```python
from build123d import *

# Parameters (mm, degrees)
BOX044_W               = 4
BOX044_H               = 7
BOX044_DEPTH           = 25
BOX044_PLACEMENT_ANGLE = 45
CYLINDER100_R          = 22
CYLINDER100_DEPTH      = 28
BOX042_W               = 26.5
BOX042_H               = 20.2
BOX042_DEPTH           = 28
BOX042_PLACEMENT_ANGLE = 45
BOX043_W               = 16.5
BOX043_H               = 36
BOX043_DEPTH           = 28
BOX043_PLACEMENT_ANGLE = 45
BOX045_W               = 10
BOX045_H               = 36
BOX045_DEPTH           = 3
BOX045_PLACEMENT_ANGLE = 45


with BuildPart() as cube023:
    # Box044 → Box044 (new body)
    with BuildSketch(Plane.XY):
        with Locations((2, 3.5)):
            Rectangle(BOX044_W, BOX044_H)
    extrude(amount=BOX044_DEPTH)


with BuildPart() as cube023_1:
    # Box044 placement: moved
    add(cube023.part.moved(Location((17, 12, -28))).rotate(Axis((17, 12, -28), (0, 0, 1)), BOX044_PLACEMENT_ANGLE))


with BuildPart() as cylinder100:
    # Cylinder100 → Cylinder100 (new body)
    with BuildSketch(Plane(origin=(7, 7, -28), x_dir=(1, 0, 0), z_dir=(0, 0, 1))):
        Circle(CYLINDER100_R)
    extrude(amount=CYLINDER100_DEPTH)


with BuildPart() as inner001:
    # Box042 → Box042 (new body)
    with BuildSketch(Plane.XY):
        with Locations((13.25, 10.1)):
            Rectangle(BOX042_W, BOX042_H)
    extrude(amount=BOX042_DEPTH)


with BuildPart() as inner001_1:
    # Box042 placement: moved
    add(inner001.part.moved(Location((24.2, 10, -28))).rotate(Axis((24.2, 10, -28), (0, 0, 1)), BOX042_PLACEMENT_ANGLE))


with BuildPart() as cut106:
    # Box043 → Box043 (new body)
    with BuildSketch(Plane.XY):
        with Locations((8.25, 18)):
            Rectangle(BOX043_W, BOX043_H)
    extrude(amount=BOX043_DEPTH)


with BuildPart() as cut106_1:
    # Box043 placement: moved
    add(cut106.part.moved(Location((27.2, 2, -28))).rotate(Axis((27.2, 2, -28), (0, 0, 1)), BOX043_PLACEMENT_ANGLE))

    # Cut105: cut inner001
    add(inner001_1.part, mode=Mode.SUBTRACT)

    # Common007: intersect Cylinder100
    add(cylinder100.part, mode=Mode.INTERSECT)

    # Cut106: cut Cube023
    add(cube023_1.part, mode=Mode.SUBTRACT)


with BuildPart() as fusion030:
    # Box045 → Box045 (new body)
    with BuildSketch(Plane.XY):
        with Locations((5, 18)):
            Rectangle(BOX045_W, BOX045_H)
    extrude(amount=BOX045_DEPTH)


with BuildPart() as fusion030_1:
    # Box045 placement: moved
    add(fusion030.part.moved(Location((20.19, -5, -3))).rotate(Axis((20.19, -5, -3), (0, 0, 1)), BOX045_PLACEMENT_ANGLE))

    # Fusion030: union Cut106
    add(cut106_1.part)


solid = fusion030_1.part
```
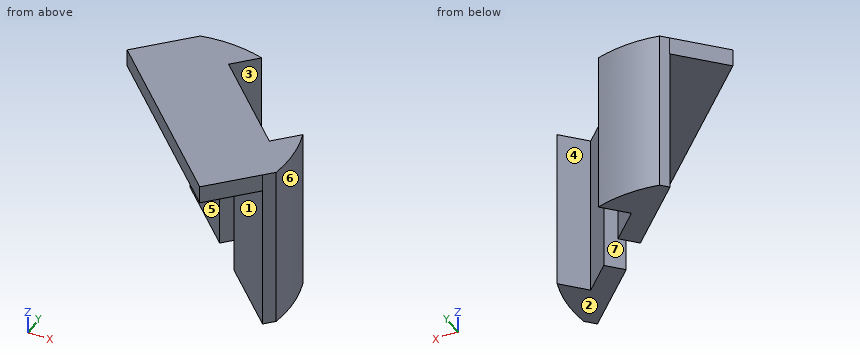
For this review, take the finished solid that the model builds, in its own axes (mm). Face numbers are marked on the shaded views. A direction names the side the tool comes from. Coordinates: 2 decimals unless noted, no trailing zeros. Write each loop counter-clockwise with the first axis right and the second up, starting at its lowest first coordinate (ties: lowest second). Pieces come first, ordered by that corner, then holes. Notation, with made-up numbers: (12, -18) - (51, -18) arc R17 ccw to (51, -9) - close; hole circle Ø6 at (78.25, 14). An arc over 180 degrees is marked (long way). Put each result on its own line as item: value.
1. Add section D-D, the plane x = 16. Give the boundary of the cut face in (y, z), then the cut area to 3 significant figures.
Values found:
outline: (-0.81, -3) - (18.2, -3) - (18.2, 0) - (-0.81, 0) - close
area: 57.0 mm²
2. Add section B-B, the plane y = 11.5. Give the boundary of the cut face in (x, z).
Values found:
outline: (3.69, -3) - (17.7, -3) - (17.7, -28) - (22.7, -28) - (22.7, 0) - (3.69, 0) - close; (25.7, -28) - (28.53, -28) - (28.53, 0) - (25.7, 0) - close
3. For pin 1 (3 mm diameter, centred on y = 20, z = -13, fed in from -X); pin 2 (8 mm diameter, centred on y = 12, z = -10.5, fed in from -X); pin 3 (1.5 mm diameter, centred on y = 16, z = -23.5, fed in from +X); pin 4 (1.5 mm diameter, centred on x = 18.5, z = -13, fed in from +Y), all flat-tipped, find the tip position at first contact; note any pin that passes through.
Values found:
pin 1: x = 7.7
pin 2: x = 17.1
pin 3: through
pin 4: y = 14.25
4. Mouldability with a two-part tool opening along Y and no side actions: class the marked faces 1, 2, 3 and 4 as released by +Y, released by -Y, zero draft, split by the parting line, or undercut.
Values found:
face 1: released by -Y
face 2: zero draft
face 3: undercut
face 4: released by +Y
5. Wall thickness on probe 1 along Z at (x, y) = (2.5, 20); probe 2 along Y at (x, z) = (10, -26.5); probe 3 along X at (y, z) = (11, -13.75): over which ranges is each line inside the solid? List them lowest first.
Values found:
probe 1: -3 to 0
probe 2: 19.2 to 24.2, 24.37 to 28.79
probe 3: 18.2 to 23.2, 25.2 to 28.63
6. Machinability: for the marked faces 5, 6 and 7, which of the approach directions +Z, -Z, +X, -X, +Y, -Y give a long, thin tool a straight path to every point of the face, cutting with its end or side? Answer none if there is none.
Values found:
face 5: -Z, -X, -Y
face 6: +Z, -Z, +X
face 7: -Z, -X, +Y
7. Add section A-A, the plane z = -20.5. Give the boundary of the cut face in (x, y), then the cut area to 3 significant figures.
Values found:
outline: (1.74, 27.46) - (12.15, 17.05) - (14.65, 19.55) - (9.92, 24.28) - (13.61, 27.98) arc R22 ccw to (2.9, 28.62) - close; (17.1, 12.1) - (27.2, 2) - (28.72, 3.52) arc R22 ccw to (27.94, 13.74) - (24.2, 10) - (19.6, 14.6) - close
area: 140 mm²
8. Add section C-C, the plane y = 3. Give the boundary of the cut face in (x, z), then the cut area to 3 significant figures.
Values found:
outline: (12.19, -3) - (26.2, -3) - (26.2, -28) - (28.2, -28) - (28.2, 0) - (12.19, 0) - close
area: 98.0 mm²
